Part model, mm, in its own coordinate system. A direction names the side the tool comes from. Give positions to 0.01 mm unless a question says otherwise; leave off trailing zeros. Order: outer loops, then holes, each group sorted by start corner. A loop starts at its lowest first (then second) coordinate and runs counter-clockwise, first axis right, second up. Notation, with made-up numbers: (26, 43) - (45, 43) arc R21 ccw to (45, 55) - close; hole circle Ø5 at (45.25, 25). An arc over 180 degrees is marked (long way). Use one line per item in the form item = value. Start each with the question number.
1. Band-saw the part on A-A, the plane y = 83.5. List the corners of the cut face in (x, z).
2. Pin check, flat tips, straight feed: P1, Ø10, axis at y = 0, z = 41.5, coming from the -X side; P2, Ø1.5, axis at x = -13.5, y = 20, coming from the +Z side; P3, Ø6, axis at y = 92.5, z = -5.5, coming from the -X side. Stop position of each tip, or through.
3. Tool access for faces 5 (the face through (-78.258, -49.953, 90.133)), 6 (the face through (37, 46.831, 68)): list every direction of +Z, -Z, +X, -X, +Y, -Y with a clear straight run to the whole face (end or side of a thin tool).
4. Pull direction X, two halves, no side cores. Call faces 1 (the face through (-66.82, 90.66, 51.24)), 2 (the face through (88.065, 91.904, -27.733)), 3 (the face through (-124.688, -67.265, 74.8)), 4 (the face through (-6.99, -59.24, 68.05)): +X half, -X half, draft (parallel to the pull), parting line (faces both ways), or undercut.
5. Drill centre lines: line 1 (Z direction, x = 3, y = 33); line 2 (X direction, y = 103, z = -67.5); line 3 (Z direction, x = -138.5, y = -53). Where is each one in solid material? Low to high.
from build123d import *

# Parameters (mm, degrees)
SKETCH3_R   = 92.329
SKETCH3_R_2 = 77.0255


with BuildPart() as part:
    # Sketch1 → Revolve1 (revolve)
    with BuildSketch(Plane.XY):
        Polygon((-30.690025294, -161.262949294), (32.171767554, -98.401156447), (26.280719538, -92.510108431), (-36.284724857, -155.668249731), align=None)
    revolve(axis=Axis((-95.976487294, -95.976487294, 0), (0.707106781, 0.707106781, 0)))



with BuildPart() as body_2:
    # Sketch2 → Revolve2 (revolve)
    with BuildSketch(Plane.XY):
        Polygon((84.4169, 135.73125), (83.9978, 46.83125), (92.329, 46.83125), (92.329, 135.73125), align=None)
    revolve(axis=Axis((0, 0, 0), (0, 1, 0)))


with BuildPart() as part_1:
    add(part.part)

    add(body_2.part)  # Sweep1 merges body 2
    # Sweep1: sweep along a path in Sketch4
    with BuildLine(Plane.XY) as sweep1_path:
        ThreePointArc((-33.114694446, -33.114694446), (-8.606228687, 3.564816643), (0, 46.83125))
    # Sketch3 → Sweep1 (sweep)
    with BuildSketch(Plane(origin=(-33.114694446, -33.114694446, 0), x_dir=(0, 0, -1), z_dir=(0.707106781, 0.707106781, 0))):
        Circle(SKETCH3_R)
        Circle(SKETCH3_R_2, mode=Mode.SUBTRACT)
    sweep(path=sweep1_path.line)


solid = part_1.part
From the geometry:
q1.outline = circle Ø184.66 at (0, 0); hole circle Ø168.34 at (0, 0)
q2.P1 = -122.69
q2.P2 = 91.87
q2.P3 = -92.3
q3.face_5 = none
q3.face_6 = +Y
q4.face_1 = undercut
q4.face_2 = parting line
q4.face_3 = -X half
q4.face_4 = undercut
q5.line_1 = -92.25 to -76.93, 76.93 to 92.25
q5.line_2 = -63 to -50.44, 50.44 to 63
q5.line_3 = -69.78 to -58.91, 58.91 to 69.78
